```python
from build123d import *

# Parameters (mm, degrees)
F0_W     = 25
F0_H     = 81
F1_DEPTH = 2
F2_W     = 20.8
F2_H     = 76.8
F2_W_2   = 16.8
F2_H_2   = 72.8
F3_DEPTH = 5


with BuildPart() as f1:
    # F0 (on Top) → F1 (new body)
    with BuildSketch(Plane.XY):
        with Locations((12.5, 40.5)):
            Rectangle(F0_W, F0_H)
    extrude(amount=-F1_DEPTH)

    # F2 (on Top) → F3 (join)
    with BuildSketch(Plane.XY):
        with Locations((12.5, 40.5)):
            Rectangle(F2_W, F2_H)
        with Locations((12.5, 40.5)):
            Rectangle(F2_W_2, F2_H_2, mode=Mode.SUBTRACT)
    extrude(amount=F3_DEPTH)


solid = f1.part
```
The model under review builds one solid part; all positions refer to its coordinate system, in mm. A direction names the side the tool comes from. Give positions to 0.01 mm unless a question says otherwise; leave off trailing zeros. Order: outer loops, then holes, each group sorted by start corner. A loop starts at its lowest first (then second) coordinate and runs counter-clockwise, first axis right, second up. Notation, with made-up numbers: (44, 48) - (59, 48) arc R29 ccw to (59, 87) - close; hole circle Ø3 at (54, -14.5). An arc over 180 degrees is marked (long way). Use CSV: the item, a comma, the result in double quotes. Start each with the question number.
Q1. We need section C-C, the plane y = 60.5. Write out the cut boundary in (x, z), and give its area (3 significant figures).
Q2. We need section B-B, the plane x = 10.75. Write out the cut boundary in (y, z).
Q3. The part is to be moulded in two halves that separate along X. For faces 6 (the flat face through (2.1, 40, 2)), 7 (the flat face through (12, 4.1, 2)), 8 (the flat face through (12, 0, -1)), say which applies: +X half, -X half, draft (parallel to the pull), parting line (faces both ways), or undercut.
Q4. We need section A-A, the plane z = 1.5. Write out the cut boundary in (x, y).
Q5. Tool access review of faces 1 (the flat face through (22.9, 40, 2)), 2 (the flat face through (12, 78.9, 2)), 3 (the flat face through (12, 41, -2)), 4 (the flat face through (12, 2.1, 2)), 5 (the flat face through (12, 76.9, 2)): name each direction out of +Z, -Z, +X, -X, +Y, -Y from which nothing blocks a thin tool from reaching the whole face with its end or side.
Q6. Clearance check with flat-ended pins moving along their axes: pin 1 Ø4 at (x, z) = (14, 3.5) entering from +Y; pin 2 Ø2.5 at (y, z) = (53.5, 3.5) entering from +X; pin 3 Ø5 at (x, y) = (15, 15.5) entering from +Z. State where each tip first meets the part, or that it passes through.
Q7. To check wall thickness, follow line 1 along Y through (x, z) = (19.25, 2.25); line 2 along X through (y, z) = (9.5, 0.5); line 3 along Z through (x, y) = (2, 4.5). State the ranges of each line that lie inside material, in increasing order. Write a range as [from, to].
Outcome:
1,outline,"(0, -2) - (25, -2) - (25, 0) - (22.9, 0) - (22.9, 5) - (20.9, 5) - (20.9, 0) - (4.1, 0) - (4.1, 5) - (2.1, 5) - (2.1, 0) - (0, 0) - close"
1,area,"70.0 mm^2"
2,outline,"(0, -2) - (81, -2) - (81, 0) - (78.9, 0) - (78.9, 5) - (76.9, 5) - (76.9, 0) - (4.1, 0) - (4.1, 5) - (2.1, 5) - (2.1, 0) - (0, 0) - close"
3,face 6,"-X half"
3,face 7,"undercut"
3,face 8,"draft"
4,outline,"(2.1, 2.1) - (22.9, 2.1) - (22.9, 78.9) - (2.1, 78.9) - close; hole (4.1, 4.1) - (20.9, 4.1) - (20.9, 76.9) - (4.1, 76.9) - close"
5,face 1,"+Z, +X, +Y, -Y"
5,face 2,"+Z, +X, -X, +Y"
5,face 3,"-Z, +X, -X, +Y, -Y"
5,face 4,"+Z, +X, -X, -Y"
5,face 5,"+Z"
6,pin 1,"stops at y = 78.9"
6,pin 2,"stops at x = 22.9"
6,pin 3,"stops at z = 0"
7,line 1,"y = [2.1, 4.1], [76.9, 78.9]"
7,line 2,"x = [2.1, 4.1], [20.9, 22.9]"
7,line 3,"z = [-2, 0]"
